Verification items for the finished model (mm, model axes). A direction names the side the tool comes from. Give positions to 0.01 mm unless a question says otherwise; leave off trailing zeros. Order: outer loops, then holes, each group sorted by start corner. A loop starts at its lowest first (then second) coordinate and runs counter-clockwise, first axis right, second up. Notation, with made-up numbers: M 33.5,2.5 L 70.5,2.5 A21 cw 70.5,38.5 Z; hole C 68,48 d1. An arc over 180 degrees is marked long. Answer as a JSON object with one key per item and string values.
```python
from build123d import *

# Parameters (mm, degrees)
BOSS_EXTRUDE2_DEPTH = 20
FILLET1_RADIUS      = 10
FILLET1_LENGTH      = 5
FILLET2_RADIUS      = 10
FILLET2_LENGTH      = 5
SKETCH5_R           = 1
SKETCH5_R_2         = 5.5
CUT_EXTRUDE5_DEPTH  = 69.007352544
CUT_EXTRUDE7_DEPTH  = 25
FILLET5_R           = 10
BOSS_EXTRUDE5_DEPTH = 60
SKETCH13_R          = 2.1
CUT_EXTRUDE8_DEPTH  = 60
CUT_EXTRUDE9_DEPTH  = 60
CUT_EXTRUDE10_DEPTH = 60
SKETCH17_R          = 2.5
BOSS_EXTRUDE6_DEPTH = 8
SKETCH18_R          = 2.5
BOSS_EXTRUDE7_DEPTH = 9
BOSS_EXTRUDE8_DEPTH = 69


with BuildPart() as part:
    # Sketch1 → Boss-Extrude2 (new body)
    with BuildSketch(Plane.XY):
        Polygon((-25, 30), (25, 30), (25, -30), (-25, -30), (-25, -25), (-20, -25), (20, -25), (20, 25), (-20, 25), (-25, 25), align=None)
    extrude(amount=BOSS_EXTRUDE2_DEPTH)

    # Fillet1: full round fillet: the end face becomes a half cylinder, R = half its width
    fillet1_face = Plane((-25, 27.5, 10), x_dir=(0, -1, 0), z_dir=(-1, 0, 0))  # on the end face: x along it, z out of the body
    fillet1_slab = fillet1_face.offset(-FILLET1_RADIUS / 2) * Box(FILLET1_LENGTH, 2 * FILLET1_RADIUS, FILLET1_RADIUS, mode=Mode.PRIVATE)  # the body's end, R deep
    fillet1_round = Plane((-15, 27.5, 10), x_dir=(-1, 0, 0), z_dir=(0, -1, 0)) * Cylinder(FILLET1_RADIUS, FILLET1_LENGTH, mode=Mode.PRIVATE)  # its axis R under the face
    add(fillet1_slab - fillet1_round, mode=Mode.SUBTRACT)

    # Fillet2: full round fillet: the end face becomes a half cylinder, R = half its width
    fillet2_face = Plane((-25, -27.5, 10), x_dir=(0, -1, 0), z_dir=(-1, 0, 0))  # on the end face: x along it, z out of the body
    fillet2_slab = fillet2_face.offset(-FILLET2_RADIUS / 2) * Box(FILLET2_LENGTH, 2 * FILLET2_RADIUS, FILLET2_RADIUS, mode=Mode.PRIVATE)  # the body's end, R deep
    fillet2_round = Plane((-15, -27.5, 10), x_dir=(-1, 0, 0), z_dir=(0, -1, 0)) * Cylinder(FILLET2_RADIUS, FILLET2_LENGTH, mode=Mode.PRIVATE)  # its axis R under the face
    add(fillet2_slab - fillet2_round, mode=Mode.SUBTRACT)

    # Sketch5 → Cut-Extrude5 (cut, through all)
    with BuildSketch(Plane(origin=(0, 30, 0), x_dir=(1, 0, 0), z_dir=(0, 1, 0))):
        with Locations(Location((-15, -3, 0), (0, 0, 180))):
            Circle(SKETCH5_R)
        with Locations(Location((-22, -10, 0), (0, 0, 180))):
            Circle(SKETCH5_R)
        with Locations(Location((-15, -17, 0), (0, 0, 180))):
            Circle(SKETCH5_R)
        with Locations(Location((-8, -10, 0), (0, 0, 180))):
            Circle(SKETCH5_R)
        with Locations(Location((-15, -10, 0), (0, 0, 180))):
            Circle(SKETCH5_R_2)
    extrude(amount=-CUT_EXTRUDE5_DEPTH, mode=Mode.SUBTRACT)

    # Sketch10 → Cut-Extrude7 (cut)
    with BuildSketch(Plane(origin=(25, 0, 0), x_dir=(0, 0, -1), z_dir=(1, 0, 0))):
        Polygon((-15, 28.180148829), (-15, -28.180148829), (-15, -30), (-20, -30), (-20, 30), (-15, 30), align=None)
        Polygon((-5, 28.180148829), (-5, -28.180148829), (-5, -30), (0, -30), (0, 30), (-5, 30), align=None)
    extrude(amount=-CUT_EXTRUDE7_DEPTH, mode=Mode.SUBTRACT)

    # Fillet5
    # the kernel refuses this fillet: 10 mm, written as the material it adds along each edge
    with BuildSketch(Plane(origin=(0, 25, 15), x_dir=(1, 0, 0), z_dir=(0, 1, 0)), Plane(origin=(0, -30, 15), x_dir=(1, 0, 0), z_dir=(0, 1, 0)), Plane(origin=(0, -25, 5), x_dir=(1, 0, 0), z_dir=(0, -1, 0))) as fillet5_piece_1:
        with BuildLine():
            CenterArc((8.660254038, -10), FILLET5_R, 90, 60)
            Line((0, -5), (-0.173205081, -4.9))
            ThreePointArc((-0.173205081, -4.9), (-0.2, -2.5), (-0.2, 0))
            Line((-0.2, 0), (0, 0.2))
            Line((0, 0.2), (8.660254038, 0.2))
            Line((8.660254038, 0.2), (8.660254038, 0))
        make_face()
    extrude(amount=5)
    with BuildSketch(Plane(origin=(0, 30, 5), x_dir=(0, 0, -1), z_dir=(0, -1, 0))) as fillet5_piece_2:
        with BuildLine():
            CenterArc((10, 8.660254038), FILLET5_R, 180, 60)
            Line((0, 8.660254038), (-0.2, 8.660254038))
            Line((-0.2, 8.660254038), (-0.2, 0))
            Line((-0.2, 0), (0, -0.2))
            ThreePointArc((0, -0.2), (2.5, -0.2), (4.9, -0.173205081))
            Line((4.9, -0.173205081), (5, 0))
        make_face()
    extrude(amount=5)

    # Sketch12 → Boss-Extrude5 (add)
    with BuildSketch(Plane.XZ.offset(30)):
        with BuildLine():
            Line((56.226298398, -3.359735054), (61.222506141, 5.302707337))
            ThreePointArc((61.222506141, 5.302707337), (43.74904955, 12.533728595), (25, 15))
            Line((25, 15), (25, 5))
            ThreePointArc((25, 5), (41.16297375, 2.873903962), (56.226298398, -3.359735054))
        make_face()
    extrude(amount=-BOSS_EXTRUDE5_DEPTH)

    # Sketch13 → Cut-Extrude8 (cut)
    with BuildSketch(Plane(origin=(2.920998947, 0, 10.910870277), x_dir=(-0.9659824633840055, 0, 0.2586075800021504), z_dir=(-0.2586075800021504, 0, -0.9659824633840055))):
        with Locations((-39.019497435, 15)):
            Circle(SKETCH13_R)
        with Locations((-39.019497435, 0)):
            Circle(SKETCH13_R)
        with Locations((-39.019497435, -15)):
            Circle(SKETCH13_R)
    extrude(amount=-CUT_EXTRUDE8_DEPTH, mode=Mode.SUBTRACT)

    # Sketch15 → Cut-Extrude9 (cut)
    with BuildSketch(Plane(origin=(0, 30, 0), x_dir=(1, 0, 0), z_dir=(0, 1, 0))):
        with BuildLine():
            Line((8.660254038, -5), (8.660254038, -15))
            ThreePointArc((8.660254038, -15), (-39.182795974, -10), (8.660254038, -5))
        make_face()
    extrude(amount=-CUT_EXTRUDE9_DEPTH, mode=Mode.SUBTRACT)

    # Sketch16 → Cut-Extrude10 (cut)
    with BuildSketch(Plane(origin=(0, 30, 0), x_dir=(1, 0, 0), z_dir=(0, 1, 0))):
        Polygon((-6.307906019, -33.220384693), (8.660254038, -15), (20.000254038, -15), (20.000254038, -5), (8.660254038, -5), (3.496355525, -1.350438774), (-14.790578774, -27.225295226), align=None)
    extrude(amount=-CUT_EXTRUDE10_DEPTH, mode=Mode.SUBTRACT)

    # Sketch17 → Boss-Extrude6 (add)
    # profile 1 of 2: a face of its own
    with BuildSketch(Plane(origin=(0, 16, 0), x_dir=(1, 0, 0), z_dir=(0, 1, 0))):
        Polygon((2.432023453, -2.661202229), (-1.062108246, -7.605177784), (-12.605177784, -23.937891754), (-14.882580853, -27.160273185), (-8.757813114, -31.488924262), (-6.307906019, -33.220384693), (7.998117102, -12.978265997), (11.006698288, -8.721313737), align=None)
        with Locations(Location((-6.090722034, -22.517234763, 0), (0, 0, 180))):
            Circle(SKETCH17_R, mode=Mode.SUBTRACT)
        with Locations(Location((-0.226842709, -14.220216066, 0), (0, 0, 180))):
            Circle(SKETCH17_R, mode=Mode.SUBTRACT)
    # profile 2 of 2: a face of its own
    with BuildSketch(Plane(origin=(0, 16, 0), x_dir=(1, 0, 0), z_dir=(0, 1, 0))):
        with BuildLine():
            Line((3.360713643, -1.347164296), (2.432023453, -2.661202229))
            Line((2.432023453, -2.661202229), (11.006698288, -8.721313737))
            Line((11.006698288, -8.721313737), (7.998117102, -12.978265997))
            ThreePointArc((7.998117102, -12.978265997), (13.960401245, -14.154569005), (20.000254038, -14.827398269))
            Line((20.000254038, -14.827398269), (20.000254038, -5))
            ThreePointArc((20.000254038, -5), (11.555844657, -3.741343444), (3.360713643, -1.347164296))
        make_face()
    extrude(amount=BOSS_EXTRUDE6_DEPTH)

    # Sketch18 → Boss-Extrude7 (add)
    with BuildSketch(Plane(origin=(0, -39, 0), x_dir=(1, 0, 0), z_dir=(0, 1, 0))):
        with BuildLine():
            Line((3.360713643, -1.347164296), (-14.882580853, -27.160273185))
            Line((-14.882580853, -27.160273185), (-6.307906019, -33.220384693))
            Line((-6.307906019, -33.220384693), (7.998117102, -12.978265997))
            ThreePointArc((7.998117102, -12.978265997), (13.960401245, -14.154569005), (20.000254038, -14.827398269))
            Line((20.000254038, -14.827398269), (20.000254038, -15))
            Line((20.000254038, -15), (25, -15))
            ThreePointArc((25, -15), (43.74904955, -12.533728595), (61.222506141, -5.302707337))
            Line((61.222506141, -5.302707337), (56.226298398, 3.359735054))
            ThreePointArc((56.226298398, 3.359735054), (41.16297375, -2.873903962), (25, -5))
            Line((25, -5), (20.000254038, -5))
            ThreePointArc((20.000254038, -5), (11.555844657, -3.741343444), (3.360713643, -1.347164296))
        make_face()
        with Locations(Location((-6.090722034, -22.517234763, 0), (0, 0, 180))):
            Circle(SKETCH18_R, mode=Mode.SUBTRACT)
        with Locations(Location((-0.226842709, -14.220216066, 0), (0, 0, 180))):
            Circle(SKETCH18_R, mode=Mode.SUBTRACT)
    extrude(amount=BOSS_EXTRUDE7_DEPTH)

    # Sketch19 → Boss-Extrude8 (add)
    with BuildSketch(Plane(origin=(0, 30, 0), x_dir=(1, 0, 0), z_dir=(0, 1, 0))):
        with BuildLine():
            Line((56.226298398, 3.359735054), (61.222506141, -5.302707337))
            ThreePointArc((61.222506141, -5.302707337), (43.74904955, -12.533728595), (25, -15))
            Line((25, -15), (20.000254038, -15))
            Line((20.000254038, -15), (20.000254038, -5))
            Line((20.000254038, -5), (25, -5))
            ThreePointArc((25, -5), (41.16297375, -2.873903962), (56.226298398, 3.359735054))
        make_face()
    extrude(amount=BOSS_EXTRUDE8_DEPTH)


solid = part.part
```
Q1. Section check D-D on x = 52. Record the cut outline in (y, z).
Resolved:
{"outline": "M -39,-1.13 L 99,-1.13 L 99,9.78 L -39,9.78 Z"}
Q2. Material ranges on L1, parallel to Y at x = -5, z = 31; L2, parallel to Z at x = 25.5, y = 83.5; L3, parallel to Z at x = 37.5, y = 44, recorded low to high.
Resolved:
{"L1": "y = -39 to -30, 16 to 24", "L2": "z = 5 to 15", "L3": "z = 3.74 to 13.91"}
Q3. Release check for a two-part mould opening along Z. For faces 1 (the face through (-8.475, 19.944, 23.268)), 2 (the face through (20, -39, 11)), 3 (the face through (58.69, 29.03, 0.91)) record: +Z half, -Z half, draft (parallel to the pull), parting line (faces both ways), or undercut.
Resolved:
{"face 1": "undercut", "face 2": "draft", "face 3": "-Z half"}
Q4. Section check A-A on x = 5. Record the cut outline in (y, z), then the cut area to 3 significant figures.
Resolved:
{"outline": "M -39,1.92 L -30,1.92 L -30,17.22 L -39,17.22 Z; M 16,1.92 L 24,1.92 L 24,17.22 L 16,17.22 Z", "area": "260 mm²"}
Q5. Section check B-B on y = 20. Record the cut outline in (x, z).
Resolved:
{"outline": "M -14.88,27.16 L 3.36,1.35 A62.7 cw 20,5 L 25,5 A62.5 cw 56.23,-3.36 L 61.22,5.3 A72.5 ccw 25,15 L 20,15 L 20,14.83 A72.5 ccw 8,12.98 L -6.31,33.22 Z; hole C -6.09,22.52 d5; hole C -0.23,14.22 d5"}
Q6. Section check C-C on x = 23. Record the cut outline in (y, z).
Resolved:
{"outline": "M -39,5 L 99,5 L 99,15 L -39,15 Z"}
Q7. Gauge pin test, flat ends, axial feed: pin 1 Ø1.5 at (x, y) = (44.5, 54.5) entering from -Z; pin 2 Ø3 at (y, z) = (46.5, 6.5) entering from -X; pin 3 Ø6 at (x, z) = (-6.09, 22.52) entering from +Y. Record the tip position at first contact, or that the pin passes through.
Resolved:
{"pin 1": "stops at z = 1.63", "pin 2": "stops at x = 20", "pin 3": "stops at y = 24"}
Q8. Tool access check on faces 4 (the face through (40.5, 15.63, 8.14)), 5 (the face through (11.673, 19.944, 3.767)), 6 (the face through (2.5, -30, 14.8)). Record the directions out of +Z, -Z, +X, -X, +Y, -Y that give a thin tool (end or side, any length) a straight path to the whole face; none if there is none.
Resolved:
{"face 4": "none", "face 5": "-Z, +Y, -Y", "face 6": "+Z, -Z, -X"}
